from build123d import *

# Parameters (mm, degrees)
SKETCH1_W           = 145
SKETCH1_H           = 50
BOSS_EXTRUDE1_DEPTH = 23.2
SKETCH2_R           = 1.75
BOSS_EXTRUDE2_DEPTH = 10
SKETCH3_R           = 1.75
BOSS_EXTRUDE3_DEPTH = 10


with BuildPart() as part:
    # Sketch1 → Boss-Extrude1 (new body)
    with BuildSketch(Plane.XY):
        with Locations((-39.629237288, 11.022245763)):
            Rectangle(SKETCH1_W, SKETCH1_H)
    extrude(amount=BOSS_EXTRUDE1_DEPTH)

    # Sketch2 → Boss-Extrude2 (add)
    with BuildSketch(Plane.ZY.offset(112.129237288)):
        with Locations(Location((4.611645571, 33.494222045, 0), (0, 0, 180))):
            Circle(SKETCH2_R)
    extrude(amount=BOSS_EXTRUDE2_DEPTH)

    # Sketch3 → Boss-Extrude3 (add)
    with BuildSketch(Plane.ZY.offset(112.129237288)):
        with Locations(Location((8.487504138, 33.421885549, 0), (0, 0, 180))):
            Circle(SKETCH3_R)
    extrude(amount=BOSS_EXTRUDE3_DEPTH)


solid = part.part
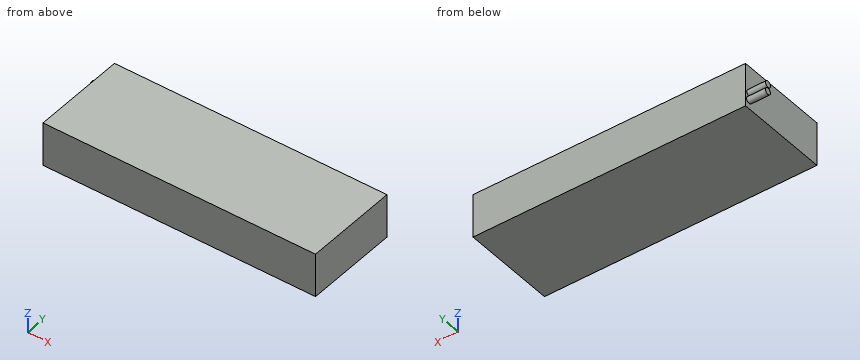
The listing builds one solid part. Answer for the finished solid, in the listing's coordinates (mm). Give positions to 0.01 mm unless a question says otherwise; leave off trailing zeros. Write each loop counter-clockwise with the first axis right and the second up, starting at its lowest first coordinate (ties: lowest second). Pieces come first, ordered by that corner, then holes.
Item 1: Section A-A, the plane z = 20.5 is taken. Write down the section's boundary in (x, y), plus the area to 3 significant figures.
Item 2: Section C-C, the plane z = 5 is taken. Write down the section's boundary in (x, y), plus the area to 3 significant figures.
Item 3: A flat-ended cylindrical pin translates along its axis: P1, Ø5, axis at y = 12.5, z = 9.5, coming from the -X side. Find the tip coordinate at first contact, or state that the pin passes through.
Item 4: Find the intervals of material crossed by line 1 along X through (y, z) = (29.5, 20.5), in increasing order.
Item 5: Section B-B, the plane y = 28 is taken. Write down the section's boundary in (x, z), plus the area to 3 significant figures.
Completed:
1. outline: (-112.13, -13.98) - (32.87, -13.98) - (32.87, 36.02) - (-112.13, 36.02) - close
1. area: 7,250 mm2
2. outline: (-122.13, 31.79) - (-112.13, 31.79) - (-112.13, -13.98) - (32.87, -13.98) - (32.87, 36.02) - (-112.13, 36.02) - (-112.13, 35.2) - (-122.13, 35.2) - close
2. area: 7,280 mm2
3. P1: stops at x = -112.13
4. line 1: x = -112.13 to 32.87
5. outline: (-112.13, 0) - (32.87, 0) - (32.87, 23.2) - (-112.13, 23.2) - close
5. area: 3,360 mm2
